Can you work these out from the model? Positions are in its coordinate system, mm. Face numbers are marked on the shaded views. Give positions to 0.01 mm unless a question says otherwise; leave off trailing zeros. Loops run counter-clockwise (first coordinate to the right, second up) from the corner with the lowest first, then second, coordinate; pieces in that order, holes last. Notation, with made-up numbers: (40, 71.25) - (93, 71.25) arc R18 ccw to (93, 97.25) - close; hole circle Ø7 at (48.25, -2.5). An arc over 180 degrees is marked (long way). Answer as a JSON object with one key per item and string values. Group by question number.
Item 1: Please list where these lines run through material, in increasing order: L1, parallel to Z at x = -892.5, y = 26.75; L2, parallel to Z at x = -484, y = -32; L3, parallel to Z at x = -905.2, y = 18.75.
Item 2: Suppose I cut it at B-B on x = -751. Write out the boundary of the cut face in (y, z), and give its area (3 significant figures).
Item 3: Will these pins go through, and if not, where does the flat tip stop? pin 1 (8 mm diameter, centred on x = -501.5, z = -113.5, fed in from +Y); pin 2 (7.5 mm diameter, centred on x = -1016, y = -34, fed in from +Z); pin 3 (17.5 mm diameter, centred on x = -895, z = 795, fed in from -Y).
Item 4: Suppose I cut it at A-A on z = 207. Write out the boundary of the cut face in (x, y).
Item 5: Thinking about a two-plate mould opening in Z: for the marked faces 1 and 2, which applies, pulls with the +Z half, pulls with the -Z half, needs draft (parallel to the pull), parting line crosses it, or undercut?
from build123d import *

# Parameters (mm, degrees)
BOSS_EXTRUDE1_DEPTH      = 1100
BOSS_EXTRUDE1_DEPTH_BACK = 300
SKETCH3_R                = 7.5
BOSS_EXTRUDE2_DEPTH      = 800
SKETCH5_R                = 7.5
CUT_EXTRUDE2_DEPTH       = 1519.191769837
SKETCH9_W                = 580
SKETCH9_H                = 60
SKETCH9_W_2              = 60
CUT_EXTRUDE5_DEPTH       = 1486.505638628
SKETCH6_W                = 25
SKETCH6_H                = 32
BOSS_EXTRUDE3_DEPTH      = 37.5
SKETCH7_W                = 16
SKETCH7_H                = 32.5
CUT_EXTRUDE3_DEPTH       = 1530.367271912
SKETCH8_W                = 16
SKETCH8_H                = 64
CUT_EXTRUDE4_DEPTH       = 24
SKETCH10_R               = 2.5908
SKETCH10_R_2             = 1.02
CUT_EXTRUDE6_DEPTH       = 20


with BuildPart() as part:
    # Sketch2 → Boss-Extrude1 (new, two sides: drawn at the far end of the back side and taken through both)
    with BuildSketch(Plane.XY.offset(-BOSS_EXTRUDE1_DEPTH_BACK)):
        Polygon((0, 0), (0, 81.865758383), (-142.5, 30), (-1042.5, 30), (-1042.5, 0), align=None)
    extrude(amount=BOSS_EXTRUDE1_DEPTH + BOSS_EXTRUDE1_DEPTH_BACK)

    # Sketch3 → Boss-Extrude2 (add)
    # profile 1 of 2: a face of its own
    with BuildSketch(Plane.XY):
        with BuildLine():
            Line((-47.5, 0), (-47.5, -50))
            ThreePointArc((-47.5, -50), (-50.428932188, -57.071067812), (-57.5, -60))
            Line((-57.5, -60), (-512.5, -60))
            ThreePointArc((-512.5, -60), (-519.571067812, -57.071067812), (-522.5, -50))
            Line((-522.5, -50), (-522.5, 0))
            Line((-522.5, 0), (-47.5, 0))
        make_face()
        with BuildLine():
            Line((-510, -42.5), (-60, -42.5))
            ThreePointArc((-60, -42.5), (-52.5, -50), (-60, -57.5))
            Line((-60, -57.5), (-510, -57.5))
            ThreePointArc((-510, -57.5), (-517.5, -50), (-510, -42.5))
        make_face(mode=Mode.SUBTRACT)
    # profile 2 of 2: a face of its own
    with BuildSketch(Plane.XY):
        with BuildLine():
            Line((-1022.5, 0), (-1022.5, -50))
            ThreePointArc((-1022.5, -50), (-1019.571067812, -57.071067812), (-1012.5, -60))
            Line((-1012.5, -60), (-1007.5, -60))
            ThreePointArc((-1007.5, -60), (-1000.428932188, -57.071067812), (-997.5, -50))
            Line((-997.5, -50), (-997.5, 0))
            Line((-997.5, 0), (-1022.5, 0))
        make_face()
        with Locations((-1010, -50)):
            Circle(SKETCH3_R, mode=Mode.SUBTRACT)
    extrude(amount=BOSS_EXTRUDE2_DEPTH)

    # Sketch5 → Cut-Extrude2 (cut, through all)
    with BuildSketch(Plane(origin=(0, 30, 0), x_dir=(1, 0, 0), z_dir=(0, 1, 0))):
        with Locations(Location((-892.5, -800, 0), (0, 0, 180))):
            Circle(SKETCH5_R)
    extrude(amount=-CUT_EXTRUDE2_DEPTH, mode=Mode.SUBTRACT)

    # Sketch9 → Cut-Extrude5 (cut, through all)
    with BuildSketch(Plane(origin=(-47.5, 0, 0), x_dir=(0, 0, -1), z_dir=(1, 0, 0))):
        with Locations((-400, -30)):
            Rectangle(SKETCH9_W, SKETCH9_H)
        Polygon((-740, -50), (-740, -60), (-800, -60), (-800, -50), (-800, 0), (-740, 0), align=None)
        with Locations((-30, -30)):
            Rectangle(SKETCH9_W_2, SKETCH9_H)
    extrude(amount=-CUT_EXTRUDE5_DEPTH, mode=Mode.SUBTRACT)

    # Sketch6 → Boss-Extrude3 (add)
    with BuildSketch(Plane.XZ):
        with Locations((-892.5, 800)):
            Rectangle(SKETCH6_W, SKETCH6_H)
    extrude(amount=BOSS_EXTRUDE3_DEPTH)

    # Sketch7 → Cut-Extrude3 (cut, through all)
    with BuildSketch(Plane.XY.offset(816)):
        with Locations((-892.5, -16.25)):
            Rectangle(SKETCH7_W, SKETCH7_H)
    extrude(amount=-CUT_EXTRUDE3_DEPTH, mode=Mode.SUBTRACT)

    # Sketch8 → Cut-Extrude4 (cut)
    with BuildSketch(Plane.XZ):
        with Locations((-892.5, 800)):
            Rectangle(SKETCH8_W, SKETCH8_H)
    extrude(amount=-CUT_EXTRUDE4_DEPTH, mode=Mode.SUBTRACT)

    # Sketch10 → Cut-Extrude6 (cut)
    with BuildSketch(Plane(origin=(0, 30, 0), x_dir=(1, 0, 0), z_dir=(0, 1, 0))):
        with Locations(Location((-892.5, 200, 0), (0, 0, 180))):
            Circle(SKETCH10_R)
        with Locations(Location((-592.5, 203.742997566, 0), (0, 0, 180))):
            Circle(SKETCH10_R)
        with Locations(Location((-292.5, 200, 0), (0, 0, 180))):
            Circle(SKETCH10_R_2)
        with Locations(Location((-905.2, -454.05, 0), (0, 0, 180))):
            Circle(SKETCH10_R)
        with Locations(Location((-879.8, -454.05, 0), (0, 0, 180))):
            Circle(SKETCH10_R)
        with Locations(Location((-605.2, -454.05, 0), (0, 0, 180))):
            Circle(SKETCH10_R)
        with Locations(Location((-579.8, -454.05, 0), (0, 0, 180))):
            Circle(SKETCH10_R)
        with Locations(Location((-305.2, -454.05, 0), (0, 0, 180))):
            Circle(SKETCH10_R)
        with Locations(Location((-279.8, -454.05, 0), (0, 0, 180))):
            Circle(SKETCH10_R)
    extrude(amount=-CUT_EXTRUDE6_DEPTH, mode=Mode.SUBTRACT)


solid = part.part
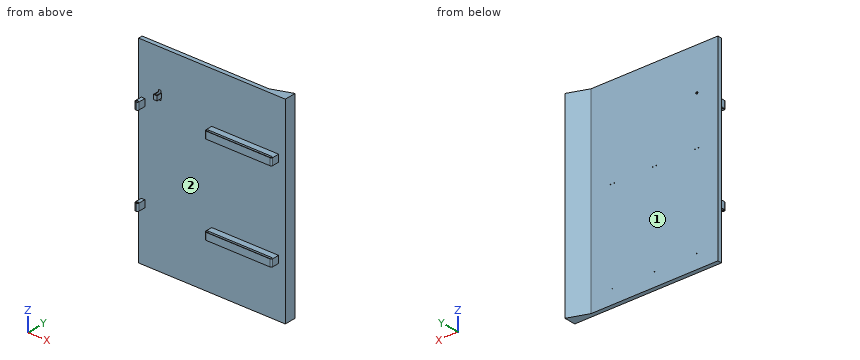
Worked out:
{
 "1": {"L1": "z = -300 to -202.59, -197.41 to 792.5, 807.5 to 1100", "L2": "z = 60 to 110, 690 to 740", "L3": "z = -300 to 451.46, 456.64 to 1100"},
 "2": {"outline": "(0, -300) - (30, -300) - (30, 1100) - (0, 1100) - close", "area": "42,000 mm2"},
 "3": {"pin 1": "stops at y = 30", "pin 2": "stops at z = 740", "pin 3": "stops at y = -37.5"},
 "4": {"outline": "(-1042.5, 0) - (0, 0) - (0, 81.87) - (-142.5, 30) - (-1042.5, 30) - close"},
 "5": {"face 1": "needs draft", "face 2": "undercut"}
}
